```python
from build123d import *

# Parameters (mm, degrees)
SKETCH1_W           = 21
SKETCH1_H           = 3
SKETCH1_W_2         = 3
SKETCH1_H_2         = 12
BOSS_EXTRUDE1_DEPTH = 3


with BuildPart() as part:
    # Sketch1 → Boss-Extrude1 (new body)
    with BuildSketch(Plane.XY):
        Polygon((-99.454545455, -7.25), (-102.454545455, -7.25), (-102.454545455, -28.75), (90.545454545, -28.75), (90.545454545, -3.75), (93.545454545, -3.75), (93.545454545, 11.25), (90.545454545, 11.25), (90.545454545, 26.25), (33.545454545, 26.25), (33.545454545, 19.25), (63.545454545, 19.25), (63.545454545, 16.25), (3.545454545, 16.25), (3.545454545, 26.25), (-72.454545455, 26.25), (-72.454545455, 19.25), (-42.454545455, 19.25), (-42.454545455, 16.25), (-102.454545455, 16.25), (-102.454545455, 4.75), (-99.454545455, 4.75), align=None)
        with Locations((-67.454545455, -20.25)):
            Rectangle(SKETCH1_W, SKETCH1_H, mode=Mode.SUBTRACT)
        with Locations((-25.454545455, -20.25)):
            Rectangle(SKETCH1_W, SKETCH1_H, mode=Mode.SUBTRACT)
        with Locations((16.545454545, -20.25)):
            Rectangle(SKETCH1_W, SKETCH1_H, mode=Mode.SUBTRACT)
        with Locations((58.545454545, -20.25)):
            Rectangle(SKETCH1_W, SKETCH1_H, mode=Mode.SUBTRACT)
        with Locations((-52.704545455, -1.25)):
            Rectangle(SKETCH1_W_2, SKETCH1_H_2, mode=Mode.SUBTRACT)
        with Locations((-4.454545455, -1.25)):
            Rectangle(SKETCH1_W_2, SKETCH1_H_2, mode=Mode.SUBTRACT)
        with Locations((43.795454545, -1.25)):
            Rectangle(SKETCH1_W_2, SKETCH1_H_2, mode=Mode.SUBTRACT)
    extrude(amount=BOSS_EXTRUDE1_DEPTH)


solid = part.part
```
Verification items for the finished model (mm, model axes). Coordinates: 2 decimals unless noted, no trailing zeros. Order: outer loops, then holes, each group sorted by start corner. A loop starts at its lowest first (then second) coordinate and runs counter-clockwise, first axis right, second up. Notation, with made-up numbers: (57.5, -2) - (76.5, -2) arc R25 ccw to (76.5, 18) - close; hole circle Ø1 at (80, -17). An arc over 180 degrees is marked (long way). Return JSON: item names as keys, results as strings.
(1) Section check C-C, the plane y = -1.5. Record the cut outline in (x, z), and give its area (3 significant figures).
Filled sheet:
{"outline": "(-99.45, 0) - (-54.2, 0) - (-54.2, 3) - (-99.45, 3) - close; (-51.2, 0) - (-5.95, 0) - (-5.95, 3) - (-51.2, 3) - close; (-2.95, 0) - (42.3, 0) - (42.3, 3) - (-2.95, 3) - close; (45.3, 0) - (93.55, 0) - (93.55, 3) - (45.3, 3) - close", "area": "552 mm^2"}
(2) Thickness scan on line 1 along X through (y, z) = (4, 1.3); line 2 along Y through (x, z) = (-58, 0.85); line 3 along Y through (x, z) = (69, 0.5). Record the ranges inside material, lowest first.
Filled sheet:
{"line 1": "x = -99.45 to -54.2, -51.2 to -5.95, -2.95 to 42.3, 45.3 to 93.55", "line 2": "y = -28.75 to -21.75, -18.75 to 16.25, 19.25 to 26.25", "line 3": "y = -28.75 to -21.75, -18.75 to 26.25"}
(3) Section check A-A, the plane x = 37.5. Record the cut outline in (y, z).
Filled sheet:
{"outline": "(-28.75, 0) - (16.25, 0) - (16.25, 3) - (-28.75, 3) - close; (19.25, 0) - (26.25, 0) - (26.25, 3) - (19.25, 3) - close"}
(4) Go/stop test with flat-tipped pins: pin 1 (1.5 mm diameter, centred on y = -21, z = 1, fed in from +X); pin 2 (1.5 mm diameter, centred on y = 18, z = 2.5, fed in from -X); pin 3 (1.5 mm diameter, centred on x = 91.5, z = 2, fed in from +Y). Record where each tip stops, or that it passes through.
Filled sheet:
{"pin 1": "stops at x = 90.55", "pin 2": "stops at x = -42.45", "pin 3": "stops at y = 11.25"}
(5) Section check D-D, the plane z = 2.05. Give the number of separate pieces and of enclosed holes in the cut face, and give its area (3 significant figures).
Filled sheet:
{"separate pieces": "1", "enclosed holes": "7", "area": "9,480 mm^2"}
(6) Section check B-B, the plane y = 21.5. Record the cut outline in (x, z), and give its area (3 significant figures).
Filled sheet:
{"outline": "(-72.45, 0) - (3.55, 0) - (3.55, 3) - (-72.45, 3) - close; (33.55, 0) - (90.55, 0) - (90.55, 3) - (33.55, 3) - close", "area": "399 mm^2"}
